Read the model definition and answer for the solid it produces. Units are mm, in the model's axes. A direction names the side the tool comes from. Give positions to 0.01 mm unless a question says otherwise; leave off trailing zeros. Write each loop counter-clockwise with the first axis right and the second up, starting at its lowest first coordinate (ties: lowest second). Pieces come first, ordered by that corner, then holes. Notation, with made-up numbers: (82, 74.25) - (119, 74.25) arc R30 ccw to (119, 106.25) - close; hole circle Ø3 at (58.5, 40.5). An arc over 180 degrees is marked (long way). Answer as CSV lines item,"result".
Autodesk Inventor part; units mm, degrees
ref_plane "YZ Plane" through (0, 0, 0) normal (1, 0, 0) x (0, 1, 0)
ref_plane "XZ Plane" through (0, 0, 0) normal (0, 1, 0) x (-1, 0, 0)
ref_plane "XY Plane" through (0, 0, 0) normal (0, 0, 1) x (1, 0, 0)
sketch "Boceto1" plane through (0, 0, 0) normal (1, 0, 0) x (0, 1, 0)
  line L0 (3, 30) -> (0, 30)
  line L1 (0, 30) -> (0, 0)
  line L2 (0, 0) -> (26.3114, -9.5766)
  line L3 (0, 0) -> (28, 0) construction
  line L4 (26.3114, -9.5766) -> (26.3114, -51.5766)
  line L5 (26.3114, -51.5766) -> (6.6152, -55.0495)
  line L6 (6.6152, -55.0495) -> (6.6152, -128.0495)
  line L7 (6.6152, -128.0495) -> (9.6152, -128.0495)
  line L8 (9.6152, -128.0495) -> (9.6152, -57.5668)
  line L9 (6.6152, -55.0495) -> (6.6152, -58.0495)
  line L10 (29.3114, -9.5766) -> (29.3114, -54.0939)
  line L11 (27.3375, -6.7575) -> (3, 2.1006)
  line L12 (3, 2.1006) -> (3, 30)
  line L13 (29.3114, -54.0939) -> (9.6152, -57.5668)
  line L14 (27.3375, -6.7575) -> (29.3114, -7.4759)
  line L15 (29.3114, -9.5766) -> (29.3114, -7.4759)
  dimension "d0" = 3
  dimension "d2" = 28
  dimension "d3" = 20
  dimension "d6" = 100
  dimension "d7" = 73
  dimension "d8" = 3
  dimension "d9" = 3
  dimension "d12" = 3
  dimension "d13" = 3
extrude "Extrusión1" add sketch "Boceto1" along normal blind 40
sketch "Boceto4" plane through (0, 9.6152, -57.5668) normal (0, 1, 0) x (1, 0, 0)
  line L0 (0, 70.4827) -> (40, 70.4827)
  line L1 (40, -2.5173) -> (40, 70.4827)
  line L2 (0, 70.4827) -> (40, 70.4827)
  line L3 (40, 70.4827) -> (40, 58.4827)
  line L4 (40, 58.4827) -> (0, 58.4827)
  line L5 (0, 58.4827) -> (0, 70.4827)
  line L6 (11, 58.4827) -> (30, 58.4827)
  line L7 (30, 58.4827) -> (30, 16.4827)
  line L8 (30, 16.4827) -> (11, 16.4827)
  line L9 (11, 16.4827) -> (11, 58.4827)
  line L10 (0, 16.4827) -> (40, 16.4827)
  line L11 (40, 16.4827) -> (40, 4.4827)
  line L12 (40, 4.4827) -> (0, 4.4827)
  line L13 (0, 4.4827) -> (0, 16.4827)
  circle A0 centre (25, 62.483) radius 1
  circle A1 centre (15, 62.483) radius 1
  circle A2 centre (25, 12.483) radius 1
  circle A3 centre (15, 12.483) radius 1
  point P0 (0, -57.5668)
  point P1 (30, 16.4827)
  dimension "d22" = 12
  dimension "d23" = 19
  dimension "d24" = 42
  dimension "d25" = 12
  dimension "d26" = 2
  dimension "d27" = 2
  dimension "d28" = 2
  dimension "d29" = 2
extrude "Extrusión4" add sketch "Boceto4" along normal blind 3 contours L0 L1 L4 L5 | L1 L12 L13 L10 L8
extrude "Extrusión5" cut sketch "Boceto4" against normal blind 3 contours A0 | A1 | A2 | A3
thread "Rosca1"
thread "Rosca2"
thread "Rosca3"
thread "Rosca4"
properties part number "1.2.4.UpperArmLink2"
(1) A cutting plane is placed at A-A (x = 11.5). Write down the section's boundary in (y, z), and give its area (3 significant figures).
Worked out:
outline,"(0, 0) - (26.31, -9.58) - (26.31, -51.58) - (6.62, -55.05) - (6.62, -128.05) - (12.62, -128.05) - (12.62, -116.05) - (9.62, -116.05) - (9.62, -74.05) - (12.62, -74.05) - (12.62, -62.05) - (9.62, -62.05) - (9.62, -57.57) - (29.31, -54.09) - (29.31, -7.48) - (27.34, -6.76) - (3, 2.1) - (3, 30) - (0, 30) - close"
area,"651 mm^2"
(2) Each of these flat-tipped pins is pushed along its axis until it touches: P1, Ø2.5, axis at x = 29.5, y = 10.5, coming from the +Z side; P2, Ø1.8, axis at x = 15, z = -70.05, coming from the -Y side; P3, Ø2, axis at x = 23.5, z = -107.5, coming from the -Y side; P4, Ø6, axis at x = 31.5, y = 25, coming from the +Z side. Where does it stop, or does it pass through?
Worked out:
P1,"stops at z = -0.17"
P2,"passes through"
P3,"stops at y = 6.62"
P4,"stops at z = -4.81"
(3) Find the intervals of material crossed by L1, parallel to Z at x = 25, y = 9.15; L2, parallel to Z at x = 15, y = 7.9; L3, parallel to Y at x = 21.5, z = 17, in increasing order.
Worked out:
L1,"z = -128.05 to -121.05, -119.05 to -71.05, -69.05 to -54.6, -3.33 to -0.14"
L2,"z = -128.05 to -121.05, -119.05 to -71.05, -69.05 to -54.82, -2.88 to 0.32"
L3,"y = 0 to 3"
(4) A cutting plane is placed at C-C (z = -42.5). Write down the section's boundary in (x, y).
Worked out:
outline,"(0, 26.31) - (40, 26.31) - (40, 29.31) - (0, 29.31) - close"
(5) The mould has two halves that part along Z. Classify faces 1 (the flat face through (20, 2, 30)), 2 (the flat face through (20, 11, -116.05)), 3 (the flat face through (0, 14, -55)): +Z half, -Z half, draft (parallel to the pull), parting line (faces both ways), or undercut.
Worked out:
face 1,"+Z half"
face 2,"undercut"
face 3,"draft"
(6) For faces 4 (the flat face through (20, 11, -62.05)), 5 (the flat face through (20, 3, 16)), 6 (the flat face through (19.72, 12.97, -4.72)), 7 (the flat face through (20, 6.615, -91)), determine the directions among +Z, -Z, +X, -X, +Y, -Y from which every point of the face is accessible in a straight line to the end or side of a thin tool.
Worked out:
face 4,"+X, -X, +Y"
face 5,"+Z, +X, -X, +Y"
face 6,"+X, -X, -Y"
face 7,"-Z, +X, -X, -Y"
(7) A cutting plane is placed at B-B (y = 20.5). Write down the section's boundary in (x, z).
Worked out:
outline,"(0, -55.65) - (40, -55.65) - (40, -52.6) - (0, -52.6) - close; (0, -7.46) - (40, -7.46) - (40, -4.27) - (0, -4.27) - close"
